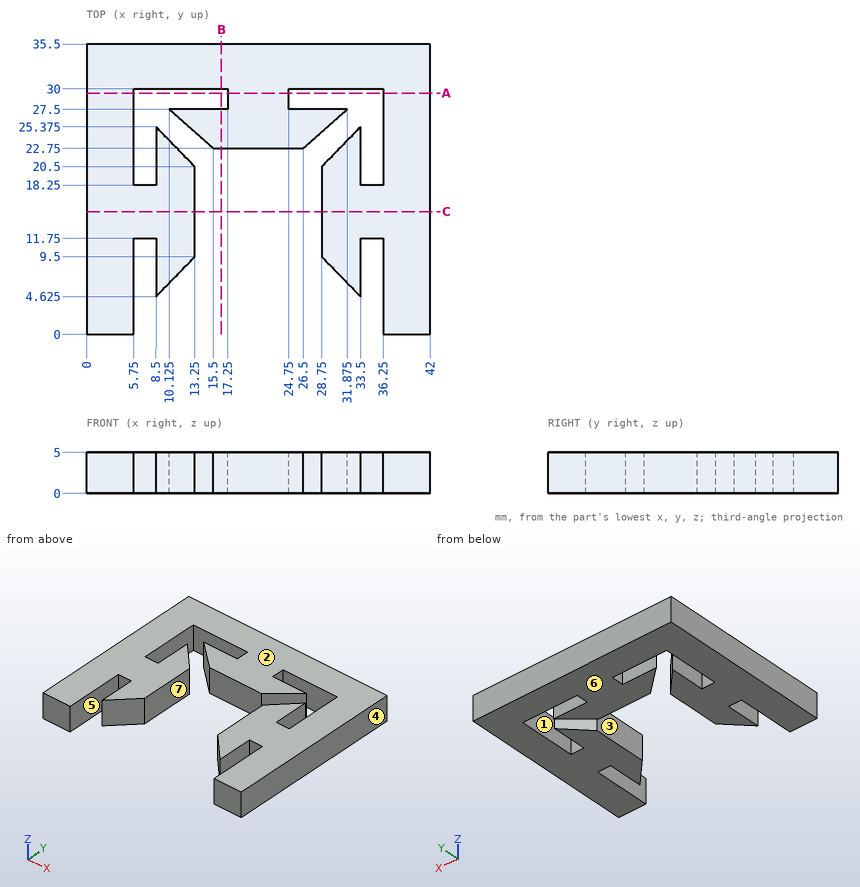
Drawing for the job (mm, zero at the part's lowest x, y, z). A direction names the side the tool comes from. Coordinates: 2 decimals unless noted, no trailing zeros. Order: outer loops, then holes, each group sorted by start corner. A loop starts at its lowest first (then second) coordinate and runs counter-clockwise, first axis right, second up.
Item 1: Band-saw the part on B-B on x = 16.5. List the corners of the cut face in (y, z).
Check sheet entries:
outline: (22.75, 0) - (27.5, 0) - (27.5, 5) - (22.75, 5) - close; (30, 0) - (35.5, 0) - (35.5, 5) - (30, 5) - close
Item 2: Pin check, flat tips, straight feed: pin 1 Ø3 at (y, z) = (29.5, 1.5) entering from -X; pin 2 Ø0.8 at (x, z) = (7, 3.5) entering from -Y. Stop position of each tip, or through.
Check sheet entries:
pin 1: stops at x = 0
pin 2: stops at y = 11.75
Item 3: Band-saw the part on A-A on y = 29.5. List the corners of the cut face in (x, z).
Check sheet entries:
outline: (0, 0) - (5.75, 0) - (5.75, 5) - (0, 5) - close; (17.25, 0) - (24.75, 0) - (24.75, 5) - (17.25, 5) - close; (36.25, 0) - (42, 0) - (42, 5) - (36.25, 5) - close
Item 4: 3-axis set-ups, long thin cutter, end or side, ignore diameter. For the marked faces 1, 2 and 3: which of +Z, -Z, +X, -X, +Y, -Y reach the whole face in a straight line?
Check sheet entries:
face 1: +Z, -Z
face 2: +Z, +X, -X, +Y, -Y
face 3: +Z, -Z, -Y
Item 5: Drill centre lines: L1, parallel to X at y = 29, z = 2.55; L2, parallel to X at y = 10.5, z = 2.45; L3, parallel to X at y = 26.5, z = 4.2. Where is each one in solid material? Low to high.
Check sheet entries:
L1: x = 0 to 5.75, 17.25 to 24.75, 36.25 to 42
L2: x = 0 to 5.75, 8.5 to 13.25, 28.75 to 33.5, 36.25 to 42
L3: x = 0 to 5.75, 11.26 to 30.74, 36.25 to 42
Item 6: Two-plate mould, pull along X, no slides. Class the marked faces 4, 5, 6 and 7: +X half, -X half, draft (parallel to the pull), parting line (faces both ways), or undercut.
Check sheet entries:
face 4: +X half
face 5: undercut
face 6: draft
face 7: undercut
Item 7: Band-saw the part on C-C on y = 15. List the corners of the cut face in (x, z).
Check sheet entries:
outline: (0, 0) - (13.25, 0) - (13.25, 5) - (0, 5) - close; (28.75, 0) - (42, 0) - (42, 5) - (28.75, 5) - close
